Input: dimensioned drawing with shaded views. Units: mm. Origin: part minimum x, y, z. Round coordinates to 2 decimals unless told otherwise and drop trailing zeros. Order: outer loops, then holes, each group sorted by start corner. A loop starts at its lowest first (then second) coordinate and runs counter-clockwise, first axis right, second up.
Item 1: Cut plane B-B on x = 28. Output: boundary loops of the cut face in (y, z), then the cut area to 3 significant figures.
Item 2: First-contact query: pin 1 (4.5 mm diameter, centred on x = 28, z = 25, fed in from -Y); pin 2 (4 mm diameter, centred on y = 3, z = 44.5, fed in from +X); pin 3 (2.5 mm diameter, centred on y = 3, z = 46, fed in from -X); pin 4 (4 mm diameter, centred on y = 3, z = 45, fed in from -X). Flat tips, straight axial feed; report the tip coordinate or a pass-through.
Item 3: Cut plane C-C on y = 3. Give the number of separate pieces and of enclosed holes in the cut face, then the cut area to 3 significant figures.
Item 4: Cut plane A-A on z = 25. Output: boundary loops of the cut face in (x, y), then the cut area to 3 significant figures.
Item 5: Line query: L1, parallel to X at y = 4.5, z = 25; L2, parallel to Z at x = 28, y = 2.5; L3, parallel to X at y = 5, z = 24. Output: solid intervals per line, ascending.
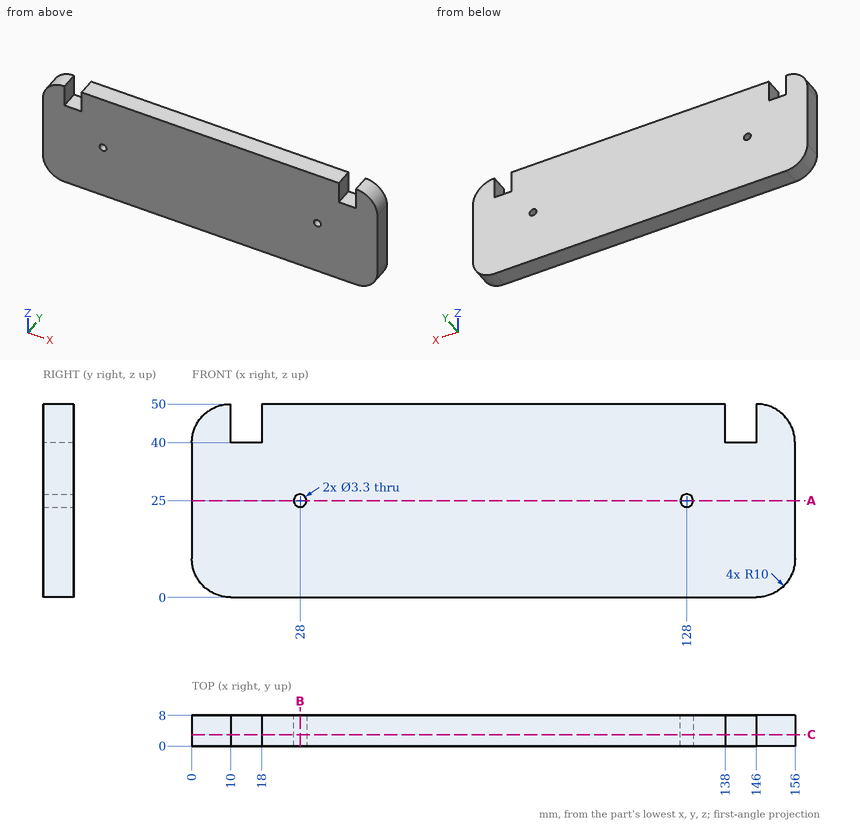
From the geometry:
1. outline: (0, 0) - (8, 0) - (8, 23.35) - (0, 23.35) - close; (0, 26.65) - (8, 26.65) - (8, 50) - (0, 50) - close
1. area: 374 mm2
2. pin 1: stops at y = 0
2. pin 2: stops at x = 155.68
2. pin 3: stops at x = 1.2
2. pin 4: stops at x = 0.46
3. separate pieces: 1
3. enclosed holes: 2
3. area: 7,540 mm2
4. outline: (0, 0) - (26.35, 0) - (26.35, 8) - (0, 8) - close; (29.65, 0) - (126.35, 0) - (126.35, 8) - (29.65, 8) - close; (129.65, 0) - (156, 0) - (156, 8) - (129.65, 8) - close
4. area: 1,200 mm2
5. L1: x = 0 to 26.35, 29.65 to 126.35, 129.65 to 156
5. L2: z = 0 to 23.35, 26.65 to 50
5. L3: x = 0 to 26.69, 29.31 to 126.69, 129.31 to 156
